Here's how the part is built. I have some questions about the finished solid (model axes, mm). A direction names the side the tool comes from. Round coordinates to 2 decimals unless told otherwise and drop trailing zeros. Loops run counter-clockwise (first coordinate to the right, second up) from the corner with the lowest first, then second, coordinate; pieces in that order, holes last. Notation, with made-up numbers: M 40,40.5 L 80,40.5 A23 ccw 80,64.5 Z; hole C 53.25,-20 d9. An arc over 180 degrees is marked long. Use a Markdown table: item, result.
Autodesk Inventor part; units mm, degrees
ref_plane "YZ Plane" through (0, 0, 0) normal (1, 0, 0) x (0, 1, 0)
ref_plane "XZ Plane" through (0, 0, 0) normal (0, 1, 0) x (-1, 0, 0)
ref_plane "XY Plane" through (0, 0, 0) normal (0, 0, 1) x (1, 0, 0)
sketch "スケッチ1" plane through (0, 0, 0) normal (0, 0, 1) x (1, 0, 0)
  line L0 (0, 5.7735) -> (5, 2.8868)
  line L1 (5, 2.8868) -> (5, -2.8868)
  line L2 (5, -2.8868) -> (0, -5.7735)
  line L3 (0, -5.7735) -> (-5, -2.8868)
  line L4 (-5, -2.8868) -> (-5, 2.8868)
  line L5 (-5, 2.8868) -> (0, 5.7735)
  circle A0 centre (0, 0) radius 1.8
  dimension "d0" = 10
  dimension "d1" = 3.6
extrude "押し出し1" add sketch "スケッチ1" along normal blind 2
sketch "スケッチ2" plane through (0, 0, 0) normal (0, 0, -1) x (-1, 0, 0)
  circle A0 centre (0, 0) radius 1.8
  circle A1 centre (0, 0) radius 4
  circle A2 centre (0, 0) radius 1.8
  dimension "d4" = 8
extrude "押し出し2" add sketch "スケッチ2" along normal blind 4
sketch "スケッチ3" plane through (0, 0, -4) normal (0, 0, -1) x (-1, 0, 0)
  circle A0 centre (0, 0) radius 3.5
  circle A1 centre (0, 0) radius 1.8
  circle A2 centre (0, 0) radius 1.8
  dimension "d7" = 7
extrude "押し出し3" add sketch "スケッチ3" along normal blind 10 contours A0 | A1
sketch "スケッチ4" plane through (0, 0, -14) normal (0, 0, -1) x (-1, 0, 0)
  line L0 (1.5, -1.5) -> (-1.5, -1.5)
  line L1 (-1.5, -1.5) -> (-1.5, 1.5)
  line L2 (-1.5, 1.5) -> (1.5, 1.5)
  line L3 (1.5, 1.5) -> (1.5, -1.5)
  line L4 (1.5, -1.5) -> (-1.5, 1.5) construction
  line L5 (-1.5, -1.5) -> (1.5, 1.5) construction
  point P0 (0, 0)
  dimension "d10" = 3
  dimension "d11" = 3
extrude "押し出し4" add sketch "スケッチ4" along normal blind 6.5
properties part number "MJ073H"
1. I need wall thicknesses on probe 1 along X at (y, z) = (0, 1.1); probe 2 along Z at (x, y) = (-1, -0.75); probe 3 along Y at (x, z) = (0.25, -0.75). Which ranges of each line are inside material? Lowest first, please. Write a range as from..to.
Answer sheet:
| item | result |
|---|---|
| probe 1 | -5..-1.8, 1.8..5 |
| probe 2 | -20.5..-4 |
| probe 3 | -3.99..-1.78, 1.78..3.99 |
2. We'd pull the mould along X, two halves only. Please class faces 5 (the face through (-2.465, -4.35, 0.986)), 6 (the face through (5, 0, 1)), 7 (the face through (0, 0, -4)), 8 (the face through (0.867, 3.905, -1.972)): +X half, -X half, draft (parallel to the pull), parting line (faces both ways), or undercut.
Answer sheet:
| item | result |
|---|---|
| face 5 | -X half |
| face 6 | +X half |
| face 7 | undercut |
| face 8 | parting line |
3. Imagine slicing it at C-C, the plane z = -3. Write out the boundary of the cut face in (x, y).
Answer sheet:
| item | result |
|---|---|
| outline | C 0,0 d8; hole C 0,0 d3.6 |
4. Imagine slicing it at D-D, the plane y = -3.25. Write out the boundary of the cut face in (x, z).
Answer sheet:
| item | result |
|---|---|
| outline | M -4.37,0 L -2.33,0 L -2.33,-4 L -1.3,-4 L -1.3,-14 L 1.3,-14 L 1.3,-4 L 2.33,-4 L 2.33,0 L 4.37,0 L 4.37,2 L -4.37,2 Z |
5. Imagine slicing it at A-A, the plane y = 0. Write out the boundary of the cut face in (x, z), then the cut area to 3 significant figures.
Answer sheet:
| item | result |
|---|---|
| outline | M -5,0 L -4,0 L -4,-4 L -3.5,-4 L -3.5,-14 L -1.5,-14 L -1.5,-20.5 L 1.5,-20.5 L 1.5,-14 L 3.5,-14 L 3.5,-4 L 4,-4 L 4,0 L 5,0 L 5,2 L 1.8,2 L 1.8,-4 L -1.8,-4 L -1.8,2 L -5,2 Z |
| area | 120 mm2 |
6. For pin 1 Ø2 at (x, y) = (1, -4.5) entering from -Z; pin 2 Ø1.5 at (x, z) = (0, -16.5) entering from +Y; pin 3 Ø1.5 at (x, z) = (-2.5, -2.5) entering from +Y, each with a flat end and sliding along its axis, tell me the tip position at first contact or that it passes through.
Answer sheet:
| item | result |
|---|---|
| pin 1 | z = -4 |
| pin 2 | y = 1.5 |
| pin 3 | y = 3.6 |
7. Which directions (+Z, -Z, +X, -X, +Y, -Y) give clear straight access to the entire face, cutting with the end or side of a thin tool? Please do faces 1 (the face through (0, -1.5, -17)), 2 (the face through (1.5, 0, -17)), 3 (the face through (0, 1.5, -17)), 4 (the face through (-3, -3, 0)).
Answer sheet:
| item | result |
|---|---|
| face 1 | -Z, +X, -X, -Y |
| face 2 | -Z, +X, +Y, -Y |
| face 3 | -Z, +X, -X, +Y |
| face 4 | -Z |
8. Imagine slicing it at B-B, the plane z = -13.25. Write out the boundary of the cut face in (x, y).
Answer sheet:
| item | result |
|---|---|
| outline | C 0,0 d7 |
